Autodesk Inventor part; units mm, degrees
ref_plane "YZ Plane" through (0, 0, 0) normal (1, 0, 0) x (0, 1, 0)
ref_plane "XZ Plane" through (0, 0, 0) normal (0, 1, 0) x (-1, 0, 0)
ref_plane "XY Plane" through (0, 0, 0) normal (0, 0, 1) x (1, 0, 0)
sketch "Sketch1" plane through (0, 0, 0) normal (0, 1, 0) x (-1, 0, 0)
  line L0 (-15, 15) -> (15, 15)
  line L1 (15, 15) -> (15, -15)
  line L2 (15, -15) -> (-15, -15)
  line L3 (-15, -15) -> (-15, 15)
  line L4 (-15, 15) -> (15, -15) construction
  line L5 (15, 15) -> (-15, -15) construction
  point P0 (0, 0)
  dimension "d0" = 30
  dimension "d1" = 30
extrude "Extrusion1" add sketch "Sketch1" along normal blind 5
sketch "Sketch2" plane through (0, 5, 0) normal (0, 1, 0) x (1, 0, 0)
  circle A0 centre (0, 0) radius 7
  dimension "d4" = 14
extrude "Extrusion2" add sketch "Sketch2" along normal blind 10
sketch "Sketch3" plane through (0, 5, 0) normal (0, 1, 0) x (1, 0, 0)
  line L0 (-15, -15) -> (15, -15)
  line L1 (0, -15) -> (0, 15) construction
  line L2 (15, 15) -> (-15, 15)
  line L3 (0, 0.1067) -> (-10, 0.1067) construction
  circle A0 centre (-10, 0.1067) radius 1.4
  point P0 (0, 0)
  point P1 (0, 0)
  dimension "d7" = 2.8
  dimension "d8" = 10
extrude "Extrusion3" add sketch "Sketch3" along normal blind 10
pattern_circular "Circular Pattern1" count 4 over 360 about axis through (0, 5, 0) along (0, 1, 0) of "Extrusion3"
sketch "Sketch4" plane through (0, 5, 0) normal (0, 1, 0) x (1, 0, 0)
  circle A0 centre (-10, 0.1067) radius 1.4
  circle A1 centre (-10, 0.1067) radius 2.5
  circle A2 centre (0.1067, 10) radius 1.4
  circle A3 centre (0.1067, 10) radius 2.5
  circle A4 centre (-0.1067, -10) radius 1.4
  circle A5 centre (-0.1067, -10) radius 2.5
  circle A6 centre (10, -0.1067) radius 1.4
  circle A7 centre (10, -0.1067) radius 2.5
  circle A8 centre (0, 0) radius 7
  circle A9 centre (0, 0) radius 8
  line L0 (15, -15) -> (-15, -15)
  line L1 (-15, -15) -> (-15, 15)
  line L2 (-15, 15) -> (15, 15)
  line L3 (15, 15) -> (15, -15)
  line L4 (15, -15) -> (-15, 15) construction
  line L5 (-15, -15) -> (15, 15) construction
  point P0 (7.8729, -1.4203)
  point P1 (1.2519, -7.9014)
  point P2 (-1.4203, -7.8729)
  point P3 (-7.9014, -1.2519)
  point P4 (-7.8729, 1.4203)
  point P5 (-1.2519, 7.9014)
  point P6 (1.4203, 7.8729)
  point P7 (7.9014, 1.2519)
  dimension "d14" = 5
  dimension "d15" = 5
  dimension "d16" = 5
  dimension "d17" = 5
  dimension "d18" = 16
extrude "Extrusion4" add sketch "Sketch4" along normal up to surface (10 mm away) contours L0 L1 L2 L3
fillet "Fillet1" radius 1 8 edges at (-1.2519, 10, -7.9014) (-7.8729, 10, -1.4203) (-7.9014, 10, 1.2519) (-1.4203, 10, 7.8729) (1.2519, 10, 7.9014) (7.8729, 10, 1.4203) (7.9014, 10, -1.2519) (1.4203, 10, -7.8729)
fillet "Fillet2" radius 2 4 edges at (15, 7.5, 15) (15, 7.5, -15) (-15, 7.5, 15) (-15, 7.5, -15)
sketch "Sketch5" plane through (-10, 15, -0.1067) normal (0, 1, 0) x (1, 0, 0)
  circle A0 centre (0, 0) radius 1.4
  circle A1 centre (0, 0) radius 1.4
  point P0 (10, -0.1067)
extrude "Extrusion5" cut sketch "Sketch5" against normal blind 20.5
pattern_circular "Circular Pattern2" count 4 over 360 about axis through (0, 5, 0) along (0, 1, 0) of "Extrusion5"
sketch "Sketch6" plane through (0, 15, 0) normal (0, 1, 0) x (1, 0, 0)
  circle A0 centre (0, 0) radius 7
  dimension "d28" = 14
extrude "Extrusion6" cut sketch "Sketch6" against normal up to surface (10 mm away)
sketch "Sketch7" plane through (0, 5, 0) normal (0, 1, 0) x (1, 0, 0)
  circle A0 centre (0, 0) radius 1.45
  dimension "d31" = 2.9
extrude "Extrusion7" cut sketch "Sketch7" against normal blind 10
equation "\"d1\" = d0"
equation "\"d15\" = d14"
equation "\"d16\" = d14"
equation "\"d17\" = d14"
properties part number "PDMS stretcher mould divided in parts"
Geometry: final body of the model. Coordinates: model frame, mm. A direction names the side the tool comes from. Give positions to 0.01 mm unless a question says otherwise; leave off trailing zeros. Loops run counter-clockwise (first coordinate to the right, second up) from the corner with the lowest first, then second, coordinate; pieces in that order, holes last. Notation, with made-up numbers: (-10.5, 17.5) - (1.5, 17.5) arc R16 ccw to (1.5, 23.5) - close; hole circle Ø4 at (-5.5, -7). An arc over 180 degrees is marked (long way). One line per question, with ' | ' between items. Start each with the question number.
(1) Section query C-C on y = 2.25. Return loops of the section in (x, z), then the cut area to 3 significant figures.
(2) Section query A-A on x = -10. Return loops of the section in (y, z), then the cut area to 3 significant figures.
(3) Ray query, line 1 (X direction, y = 1, z = 0); line 2 (Z direction, x = -10, y = 1.6); line 3 (Z direction, x = -10, y = 8.25). Return the intervals inside material, ascending. Write a range as from..to.
(4) Section query B-B on z = 10. Return loops of the section in (x, y), then the cut area to 3 significant figures.
(5) Contact query for a flat-ended pin moving along its axis: pin 1 (3 mm diameter, centred on x = 10, z = 0.11, fed in from +Y). Output: stop coordinate, or through.
(6) Pull-direction query (Z, two-part tool) for faces 1 (the cylindrical face through (-5.63, 9.93, -5.683)), 2 (the cylindrical face through (14.43, 7.6, -14.4)), 3 (the cylindrical face through (0.1, 9.9, -12.5)), 4 (the flat face through (-15, 7, 0)); classes: released by +Z, released by -Z, zero draft, split by the parting line, or undercut.
(7) Reachability of faces 5 (the cylindrical face through (5.63, 9.93, 5.683)), 6 (the cylindrical face through (-14.43, 7.4, -14.4)) from +Z, -Z, +X, -X, +Y, -Y: full face, straight path, thin tool, end or side. Return the list, or none.
(8) Section query D-D on z = -0.5. Return loops of the section in (x, y), then the cut area to 3 significant figures.
The answers:
1) outline: (-15, -13) arc R2 ccw to (-13, -15) - (13, -15) arc R2 ccw to (15, -13) - (15, 13) arc R2 ccw to (13, 15) - (-13, 15) arc R2 ccw to (-15, 13) - close; hole circle Ø2.8 at (-10, -0.11); hole circle Ø2.8 at (-0.11, 10); hole circle Ø2.9 at (0, 0); hole circle Ø2.8 at (0.11, -10); hole circle Ø2.8 at (10, 0.11) | area: 865 mm2
2) outline: (0, -15) - (15, -15) - (15, -2.61) - (5, -2.61) - (5, -1.51) - (0, -1.51) - close; (0, 1.29) - (5, 1.29) - (5, 2.39) - (15, 2.39) - (15, 15) - (0, 15) - close | area: 386 mm2
3) line 1: -15..-11.4, -8.6..-1.45, 1.45..8.6, 11.4..15 | line 2: -15..-1.51, 1.29..15 | line 3: -15..-2.61, 2.39..15
4) outline: (-15, 0) - (-1.51, 0) - (-1.51, 5) - (-2.61, 5) - (-2.61, 15) - (-15, 15) - close; (1.29, 0) - (15, 0) - (15, 15) - (2.39, 15) - (2.39, 5) - (1.29, 5) - close | area: 386 mm2
5) pin 1: y = 5
6) face 1: undercut | face 2: released by -Z | face 3: undercut | face 4: zero draft
7) face 5: +Y | face 6: -Z, -X, +Y, -Y
8) outline: (-15, 0) - (-11.34, 0) - (-11.34, 5) - (-12.47, 5) - (-12.47, 15) - (-15, 15) - close; (-8.66, 0) - (-1.36, 0) - (-1.36, 5) - (-8.66, 5) - close; (1.36, 0) - (8.74, 0) - (8.74, 5) - (1.36, 5) - close; (11.26, 0) - (15, 0) - (15, 15) - (12.43, 15) - (12.43, 5) - (11.26, 5) - close | area: 161 mm2
